```python
from build123d import *

# Parameters (mm, degrees)
F0_R     = 18.931499
F1_DEPTH = 76.2
F4_D     = 38.1
F4_DEPTH = 50.8
F5_D     = 15.875
F5_DEPTH = 50.8


with BuildPart() as f1:
    # F0 (on Front) → F1 (new body)
    with BuildSketch(Plane.XZ):
        with BuildLine():
            Line((0, -152.4), (0, 0))
            ThreePointArc((0, 0), (-76.2, -76.2), (0, -152.4))
        make_face()
        Polygon((149.225, 0), (0, 0), (0, -152.4), (149.225, -152.4), (149.225, -101.6), (73.025, -101.6), (73.025, -50.8), (149.225, -50.8), align=None)
        with Locations((34.925, -76.2)):
            Circle(F0_R, mode=Mode.SUBTRACT)
    extrude(amount=F1_DEPTH)

    # F4
    with Locations(Plane(origin=(0, 0, -50.8), x_dir=(1, 0, 0), z_dir=(0, 0, -1))):
        with Locations((111.125, 38.1)):
            Hole(F4_D / 2, depth=F4_DEPTH)

    # F5
    with Locations(Plane.XY.offset(-101.6)):
        with Locations((111.125, -38.1)):
            Hole(F5_D / 2, depth=F5_DEPTH)


solid = f1.part
```
Can you work these out from the model? Positions are in its coordinate system, mm. A direction names the side the tool comes from. Coordinates: 2 decimals unless noted, no trailing zeros. Loops run counter-clockwise (first coordinate to the right, second up) from the corner with the lowest first, then second, coordinate; pieces in that order, holes last. Notation, with made-up numbers: M 19.5,54.5 L 74.5,54.5 A31 ccw 74.5,88.5 Z; hole C 72,-38 d3. An arc over 180 degrees is marked long. Put each result on its own line as item: value. Start each with the question number.
(1) Imagine slicing it at B-B on y = -49.5. List the corners of the cut face in (x, z) for me (1 decimal).
(2) I need wall thicknesses on probe 1 along Z at (x, y) = (73.5, -15); probe 2 along Z at (x, y) = (114.5, -56.5); probe 3 along X at (y, z) = (-13.5, -76) (3 decimals). Which ranges of each line are inside material? Lowest first, please.
(3) Imagine slicing it at D-D on x = 45. List the corners of the cut face in (y, z) for me.
(4) Will these pins go through, and if not, where does the flat tip stop? pin 1 Ø1.5 at (y, z) = (-50, -82.5) entering from -X; pin 2 Ø5 at (y, z) = (-23.5, -85) entering from +X (3 decimals); pin 3 Ø2 at (y, z) = (-8, -19.5) entering from -X; pin 4 Ø1.5 at (x, y) = (31.5, -39) entering from +Z.
(5) Imagine slicing it at C-C on z = -76.2. List the corners of the cut face in (x, y) for me (1 decimal), and give its area (3 significant figures).
(6) Which directions (+Z, -Z, +X, -X, +Y, -Y) give clear straight access to the entire face, cutting with the end or side of a thin tool? Please do faces 1 (the face through (102, -21, -50.8)), 2 (the face through (20.97, -37.57, -63.41)).
(7) We'd pull the mould along X, two halves only. Please class faces 3 (the face through (115.25, -19.5, -25.04)), 4 (the face through (-76.18, -37.57, -74.52)), 5 (the face through (74, -38, -152.4)): +X half, -X half, draft (parallel to the pull), parting line (faces both ways), or undercut.
(8) Imagine slicing it at A-A on y = -38.1. List the corners of the cut face in (x, z) for me (1 decimal).
Worked answers:
1. outline: M 0,-152.4 L 149.2,-152.4 L 149.2,-101.6 L 73,-101.6 L 73,-50.8 L 95.9,-50.8 L 95.9,0 L 0,0 A76.2 ccw Z; M 126.4,-50.8 L 149.2,-50.8 L 149.2,0 L 126.4,0 Z; hole C 34.9,-76.2 d37.9
2. probe 1: z = -152.4 to -101.6, -50.8 to 0
2. probe 2: z = -152.4 to -101.6
2. probe 3: x = -76.2 to 15.995, 53.855 to 73.025
3. outline: M -76.2,-152.4 L 0,-152.4 L 0,-92.23 L -76.2,-92.23 Z; M -76.2,-60.17 L 0,-60.17 L 0,0 L -76.2,0 Z
4. pin 1: stops at x = -76
4. pin 2: stops at x = 73.025
4. pin 3: stops at x = -52
4. pin 4: stops at z = 0
5. outline: M -76.2,-76.2 L 16,-76.2 L 16,0 L -76.2,0 Z; M 53.9,-76.2 L 73,-76.2 L 73,0 L 53.9,0 Z
5. area: 8,490 mm2
6. face 1: +X, +Y, -Y
6. face 2: +Y, -Y
7. face 3: undercut
7. face 4: -X half
7. face 5: draft
8. outline: M 0,-152.4 L 103.2,-152.4 L 103.2,-101.6 L 73,-101.6 L 73,-50.8 L 92.1,-50.8 L 92.1,0 L 0,0 A76.2 ccw Z; M 119.1,-152.4 L 149.2,-152.4 L 149.2,-101.6 L 119.1,-101.6 Z; M 130.2,-50.8 L 149.2,-50.8 L 149.2,0 L 130.2,0 Z; hole C 34.9,-76.2 d37.9
